Source: CAD feature listing. Evaluate the final solid. Frame: model axes, mm. Face numbers are marked on the shaded views. A direction names the side the tool comes from. Give positions to 0.01 mm unless a question says otherwise; leave off trailing zeros. Loops run counter-clockwise (first coordinate to the right, second up) from the corner with the lowest first, then second, coordinate; pieces in that order, holes last. Notation, with made-up numbers: M 55.25,35.5 L 95.25,35.5 A27 ccw 95.25,66.5 Z; hole C -4,19 d3. An arc over 180 degrees is marked long. Put each result on its own line as item: value.
from build123d import *

# Parameters (mm, degrees)
SKETCH1_W                      = 26.08
SKETCH1_H                      = 55.016744186
SKETCH1_W_2                    = 21
SKETCH1_H_2                    = 51
BOSS_EXTRUDE1_DEPTH            = 21
SKETCH3_W                      = 26.08
SKETCH3_H                      = 2.54
BOSS_EXTRUDE2_DEPTH            = 55.016744
CUT_EXTRUDE1_REACH             = 40.482
SKETCH4_W                      = 16.428
SKETCH4_H                      = 21.016744186
CUT_EXTRUDE2_REACH             = 40.482
SKETCH5_R                      = 2.5
CUT_EXTRUDE2_DIRECTION_2_REACH = 40.482


with BuildPart() as part:
    # Sketch1 → Boss-Extrude1 (new body)
    with BuildSketch(Plane(origin=(0, 0, 0), x_dir=(1, 0, 0), z_dir=(0, 1, 0))):
        Rectangle(SKETCH1_W, SKETCH1_H)
        Rectangle(SKETCH1_W_2, SKETCH1_H_2, mode=Mode.SUBTRACT)
    extrude(amount=BOSS_EXTRUDE1_DEPTH)

    # Sketch3 → Boss-Extrude2 (add, through all)
    with BuildSketch(Plane.XY.offset(27.508372093)):
        with Locations((0, 22.27)):
            Rectangle(SKETCH3_W, SKETCH3_H)
    extrude(amount=-BOSS_EXTRUDE2_DEPTH)

    # Sketch4 → Cut-Extrude1 (cut, up to next)
    with BuildSketch(Plane(origin=(0, 23.54, 0), x_dir=(1, 0, 0), z_dir=(0, 1, 0)), mode=Mode.PRIVATE) as cut_extrude1_sk1:
        Rectangle(SKETCH4_W, SKETCH4_H)
    cut_extrude1_tool1 = extrude(cut_extrude1_sk1.sketch, amount=-CUT_EXTRUDE1_REACH, mode=Mode.PRIVATE) & part.part
    add(cut_extrude1_tool1.solids().sort_by_distance((0, 23.54, 0))[0], mode=Mode.SUBTRACT)

    # Sketch5 → Cut-Extrude2 (cut, up to next)
    with BuildSketch(Plane(origin=(0, 0, 0), x_dir=(0, 0, -1), z_dir=(1, 0, 0)), mode=Mode.PRIVATE) as cut_extrude2_sk1:
        with Locations((-9.968372093, 5.8)):
            Circle(SKETCH5_R)
    cut_extrude2_tool1 = extrude(cut_extrude2_sk1.sketch, amount=-CUT_EXTRUDE2_REACH, mode=Mode.PRIVATE) & part.part
    # Sketch5 → Cut-Extrude2 (cut, up to next)
    with BuildSketch(Plane(origin=(0, 0, 0), x_dir=(0, 0, -1), z_dir=(1, 0, 0)), mode=Mode.PRIVATE) as cut_extrude2_sk2:
        with Locations((9.968372093, 5.8)):
            Circle(SKETCH5_R)
    cut_extrude2_tool2 = extrude(cut_extrude2_sk2.sketch, amount=-CUT_EXTRUDE2_REACH, mode=Mode.PRIVATE) & part.part
    add(cut_extrude2_tool1.solids().sort_by_distance((0, 5.8, 9.968372))[0], mode=Mode.SUBTRACT)
    add(cut_extrude2_tool2.solids().sort_by_distance((0, 5.8, -9.968372))[0], mode=Mode.SUBTRACT)

    # Sketch5 → Cut-Extrude2 direction 2 (cut, up to next)
    with BuildSketch(Plane(origin=(0, 0, 0), x_dir=(0, 0, -1), z_dir=(1, 0, 0)), mode=Mode.PRIVATE) as cut_extrude2_direction_2_sk1:
        with Locations((-9.968372093, 5.8)):
            Circle(SKETCH5_R)
    cut_extrude2_direction_2_tool1 = extrude(cut_extrude2_direction_2_sk1.sketch, amount=CUT_EXTRUDE2_DIRECTION_2_REACH, mode=Mode.PRIVATE) & part.part
    # Sketch5 → Cut-Extrude2 direction 2 (cut, up to next)
    with BuildSketch(Plane(origin=(0, 0, 0), x_dir=(0, 0, -1), z_dir=(1, 0, 0)), mode=Mode.PRIVATE) as cut_extrude2_direction_2_sk2:
        with Locations((9.968372093, 5.8)):
            Circle(SKETCH5_R)
    cut_extrude2_direction_2_tool2 = extrude(cut_extrude2_direction_2_sk2.sketch, amount=CUT_EXTRUDE2_DIRECTION_2_REACH, mode=Mode.PRIVATE) & part.part
    add(cut_extrude2_direction_2_tool1.solids().sort_by_distance((0, 5.8, 9.968372))[0], mode=Mode.SUBTRACT)
    add(cut_extrude2_direction_2_tool2.solids().sort_by_distance((0, 5.8, -9.968372))[0], mode=Mode.SUBTRACT)


solid = part.part
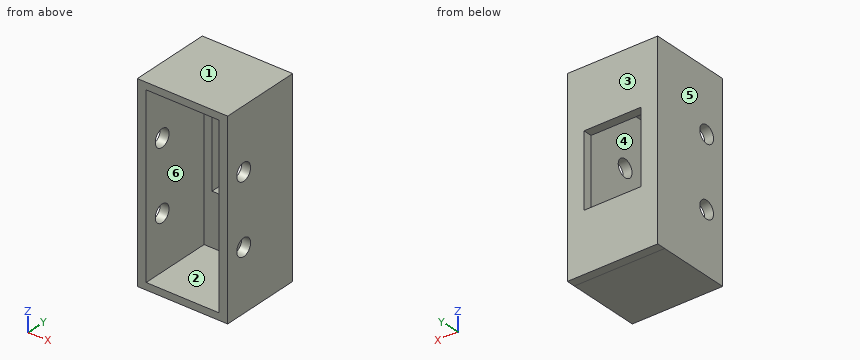
1. Contact query for a flat-ended pin moving along its axis: P1, Ø6.5, axis at x = 0, z = 6, coming from the -Y side. Output: stop coordinate, or through.
Found:
P1: through
2. Section query C-C (x = -9.5). Output: boundary loops of the cut face in (y, z).
Found:
outline: M 0,-27.51 L 23.54,-27.51 L 23.54,27.51 L 0,27.51 L 0,25.5 L 21,25.5 L 21,-25.5 L 0,-25.5 Z
3. Access query for the marked faces 1 and 2. Directions: +Z, -Z, +X, -X, +Y, -Y. A direction counts if a zero-diameter tool reaches every point of the face in a straight line with its end or side. Return the directions, or none.
Found:
face 1: +Z, +X, -X, +Y, -Y
face 2: -Y
4. Section query A-A (y = 5.8). Output: boundary loops of the cut face in (x, z).
Found:
outline: M -13.04,-27.51 L 13.04,-27.51 L 13.04,-12.47 L 10.5,-12.47 L 10.5,-25.5 L -10.5,-25.5 L -10.5,-12.47 L -13.04,-12.47 Z; M -13.04,-7.47 L -10.5,-7.47 L -10.5,7.47 L -13.04,7.47 Z; M -13.04,12.47 L -10.5,12.47 L -10.5,25.5 L 10.5,25.5 L 10.5,12.47 L 13.04,12.47 L 13.04,27.51 L -13.04,27.51 Z; M 10.5,-7.47 L 13.04,-7.47 L 13.04,7.47 L 10.5,7.47 Z
5. Section query B-B (z = 17). Output: boundary loops of the cut face in (x, y).
Found:
outline: M -13.04,0 L -10.5,0 L -10.5,21 L 10.5,21 L 10.5,0 L 13.04,0 L 13.04,23.54 L -13.04,23.54 Z
6. Draft query along X for the marked faces 3, 4, 5 and 6. Return one class per face: pulls with the +X half, pulls with the -X half, needs draft (parallel to the pull), parting line crosses it, or undercut.
Found:
face 3: needs draft
face 4: undercut
face 5: pulls with the -X half
face 6: undercut
7. Section query D-D (y = 12.25). Output: boundary loops of the cut face in (x, z), plus the area to 3 significant figures.
Found:
outline: M -13.04,-27.51 L 13.04,-27.51 L 13.04,27.51 L -13.04,27.51 Z; hole M -10.5,-25.5 L 10.5,-25.5 L 10.5,25.5 L -10.5,25.5 Z
area: 364 mm^2
8. Material intervals for line 1 (Z direction, x = 12.5, y = 5.8); line 2 (Z direction, x = 2, y = 1); line 3 (X direction, y = 6, z = 18), sorted ascending. Write a range as from..to.
Found:
line 1: -27.51..-12.47, -7.47..7.47, 12.47..27.51
line 2: -27.51..-25.5, 25.5..27.51
line 3: -13.04..-10.5, 10.5..13.04
